Geometry: see drawing. Coordinates: mm, zero at the bounding-box minimum. Coordinates: 2 decimals unless noted, no trailing zeros. Loops run counter-clockwise (first coordinate to the right, second up) from the corner with the lowest first, then second, coordinate; pieces in that order, holes last. Notation, with made-up numbers: (80, 87.5) -> (99, 87.5) arc R19 ccw to (99, 93.5) -> close; hole circle Ø1 at (31, 80.5). An arc over 180 degrees is marked (long way). One line per item, written item: value. Start each with the question number.
Item 1: Ray query, probe 1 along Y at (x, z) = (50, 1.25); probe 2 along X at (y, z) = (23, 0.7) (1 decimal); probe 3 along X at (y, z) = (24, 0.85) (1 decimal). Return the intervals inside material, ascending. Write a range as from..to.
Item 2: Section query B-B on x = 7. Return loops of the section in (y, z).
Item 3: Section query A-A on x = 50. Return loops of the section in (y, z).
Item 4: Contact query for flat-ended pins moving along their axis: pin 1 Ø2.5 at (x, y) = (35.86, 35.29) entering from +Z; pin 2 Ø1 at (x, z) = (65, 1) entering from -Y. Output: stop coordinate, or through.
Item 5: Section query D-D on y = 39. Return loops of the section in (x, z), then the cut area to 3 significant figures.
Item 6: Section query C-C on x = 94. Return loops of the section in (y, z).
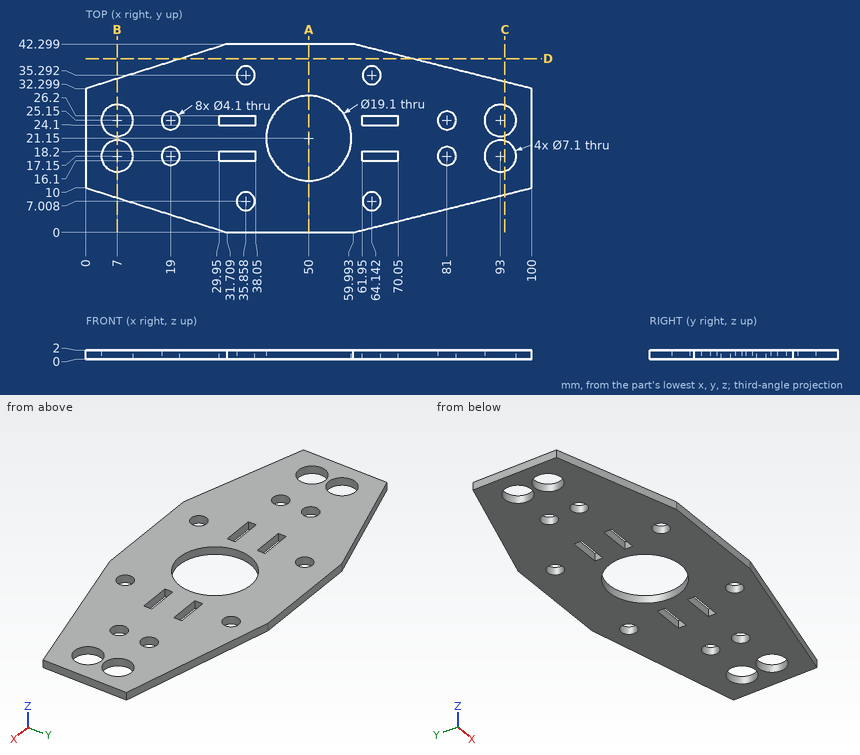
Reply:
1. probe 1: y = 0..11.6, 30.7..42.3
1. probe 2: x = 0..4.2, 9.8..40.6, 59.4..90.2, 95.8..100
1. probe 3: x = 0..3.6, 10.4..17.3, 20.7..40.9, 59.1..79.3, 82.7..89.6, 96.4..100
2. outline: (7.79, 0) -> (13.6, 0) -> (13.6, 2) -> (7.79, 2) -> close; (20.7, 0) -> (21.6, 0) -> (21.6, 2) -> (20.7, 2) -> close; (28.7, 0) -> (34.51, 0) -> (34.51, 2) -> (28.7, 2) -> close
3. outline: (0, 0) -> (11.6, 0) -> (11.6, 2) -> (0, 2) -> close; (30.7, 0) -> (42.3, 0) -> (42.3, 2) -> (30.7, 2) -> close
4. pin 1: passes through
4. pin 2: stops at y = 1.13
5. outline: (21.25, 0) -> (73.19, 0) -> (73.19, 2) -> (21.25, 2) -> close
5. area: 104 mm²
6. outline: (8.5, 0) -> (13.74, 0) -> (13.74, 2) -> (8.5, 2) -> close; (20.56, 0) -> (21.74, 0) -> (21.74, 2) -> (20.56, 2) -> close; (28.56, 0) -> (33.8, 0) -> (33.8, 2) -> (28.56, 2) -> close
